Verification items for the finished model (mm, model axes). Round coordinates to 2 decimals unless told otherwise and drop trailing zeros. Order: outer loops, then holes, each group sorted by start corner. A loop starts at its lowest first (then second) coordinate and runs counter-clockwise, first axis right, second up. Notation, with made-up numbers: M 68,-31.5 L 127,-31.5 A25 ccw 127,-7.5 Z; hole C 66.5,-20.5 d11. An arc over 180 degrees is marked long. One line per item, written item: value. Start each with the question number.
from build123d import *

# Parameters (mm, degrees)
SKETCH2_W              = 127
SKETCH2_H              = 127
BOSS_EXTRUDE1_DEPTH    = 12.7
F_10_0MM_DOWEL_HOLE1_D = 8.382
SKETCH12_R             = 7.874
CUT_EXTRUDE2_DEPTH     = 13.7


with BuildPart() as part:
    # Sketch2 → Boss-Extrude1 (new body)
    with BuildSketch(Plane(origin=(0, 0, 0), x_dir=(1, 0, 0), z_dir=(0, 1, 0))):
        Rectangle(SKETCH2_W, SKETCH2_H)
    extrude(amount=BOSS_EXTRUDE1_DEPTH)

    # Ø10.0mm Dowel Hole1 (through all)
    with Locations(Plane(origin=(0, 0, 0), x_dir=(-1, 0, 0), z_dir=(0, -1, 0))):
        with Locations((-44.45, 43.18), (-44.45, -4.572), (-44.45, -42.672), (44.45, 43.18), (44.45, -4.572), (44.45, -42.672)):
            Hole(F_10_0MM_DOWEL_HOLE1_D / 2)

    # Sketch12 → Cut-Extrude2 (cut, through all)
    with BuildSketch(Plane.XZ):
        Circle(SKETCH12_R)
    extrude(amount=-CUT_EXTRUDE2_DEPTH, mode=Mode.SUBTRACT)


solid = part.part
1. Section check D-D (y = 6). Record the cut outline in (x, z), and give its area (3 significant figures).
2. Section check A-A (z = -43.18). Record the cut outline in (x, y).
3. Scan lines: line 1 along Z through (x, y) = (44.45, 6.5); line 2 along X through (y, z) = (11.5, 43); line 3 along X through (y, z) = (5.5, 44.5). Record each from-to range of solid material in increasing order.
4. Draft check along Z on faces 1 (the face through (-47.776, 6.439, -40.63)), 2 (the face through (-1, 6, 63.5)), 3 (the face through (41.124, 6.439, -40.63)), 4 (the face through (-63.5, 6, 1)). Enter one of: released by +Z, released by -Z, zero draft, split by the parting line, or undercut.
5. Section check C-C (x = -44.45). Record the cut outline in (y, z), and give its area (3 significant figures).
6. Depth check by flat-ended pin: pin 1 (10 mm diameter, centred on x = -40.5, z = -9.5, fed in from -Y). Enter the tip coordinate at first touch or a pass-through.
7. Section check B-B (x = 0). Record the cut outline in (y, z).
Geometry check:
1. outline: M -63.5,-63.5 L 63.5,-63.5 L 63.5,63.5 L -63.5,63.5 Z; hole C -44.45,-43.18 d8.38; hole C -44.45,4.57 d8.38; hole C -44.45,42.67 d8.38; hole C 0,0 d15.75; hole C 44.45,-43.18 d8.38; hole C 44.45,4.57 d8.38; hole C 44.45,42.67 d8.38
1. area: 15,600 mm²
2. outline: M -63.5,0 L -48.64,0 L -48.64,12.7 L -63.5,12.7 Z; M -40.26,0 L 40.26,0 L 40.26,12.7 L -40.26,12.7 Z; M 48.64,0 L 63.5,0 L 63.5,12.7 L 48.64,12.7 Z
3. line 1: z = -63.5 to -47.37, -38.99 to 0.38, 8.76 to 38.48, 46.86 to 63.5
3. line 2: x = -63.5 to -48.63, -40.27 to 40.27, 48.63 to 63.5
3. line 3: x = -63.5 to -48.22, -40.68 to 40.68, 48.22 to 63.5
4. face 1: undercut
4. face 2: released by +Z
4. face 3: undercut
4. face 4: zero draft
5. outline: M 0,-63.5 L 12.7,-63.5 L 12.7,-47.37 L 0,-47.37 Z; M 0,-38.99 L 12.7,-38.99 L 12.7,0.38 L 0,0.38 Z; M 0,8.76 L 12.7,8.76 L 12.7,38.48 L 0,38.48 Z; M 0,46.86 L 12.7,46.86 L 12.7,63.5 L 0,63.5 Z
5. area: 1,290 mm²
6. pin 1: stops at y = 0
7. outline: M 0,-63.5 L 12.7,-63.5 L 12.7,-7.87 L 0,-7.87 Z; M 0,7.87 L 12.7,7.87 L 12.7,63.5 L 0,63.5 Z
